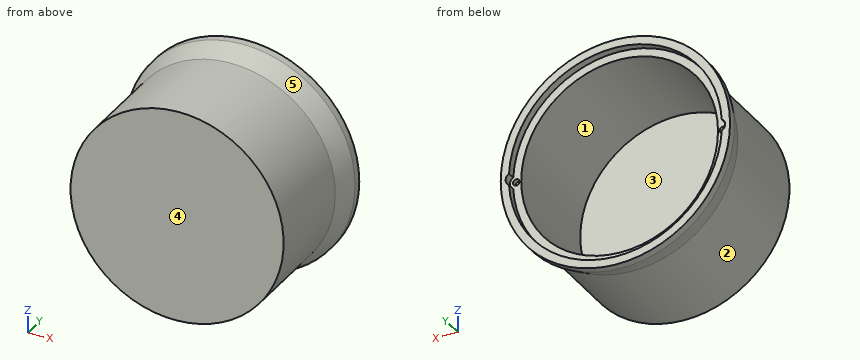
from build123d import *

# Parameters (mm, degrees)
SKETCH2_R          = 4
SKETCH2_R_2        = 2
CUT_EXTRUDE1_DEPTH = 125.761772992
SKETCH2_4_R        = 2
CUT_EXTRUDE3_DEPTH = 3


with BuildPart() as part:
    # Sketch1 → Revolve1 (revolve)
    with BuildSketch(Plane.XY, mode=Mode.PRIVATE) as revolve1_sk:
        Polygon((-70.5, 80), (-70.5, 75), (-65.5, 61.262612903), (-65.5, 0), (0, 0), (0, 5), (-60.5, 5), (-60.5, 75), (-65.5, 75), (-65.5, 80), align=None)
    revolve(revolve1_sk.sketch.rotate(Axis((0, 5, 0), (0, -1, 0)), 270), axis=Axis((0, 5, 0), (0, -1, 0)))

    # Sketch2 → Cut-Extrude1 (cut, through all)
    # profile 1 of 2: a face of its own
    with BuildSketch(Plane(origin=(0, 75, 0), x_dir=(1, 0, 0), z_dir=(0, 1, 0))):
        with Locations((-63.5, 0)):
            Circle(SKETCH2_R)
        with Locations((-63.5, 0)):
            Circle(SKETCH2_R_2, mode=Mode.SUBTRACT)
    # profile 2 of 2: a face of its own
    with BuildSketch(Plane(origin=(0, 75, 0), x_dir=(1, 0, 0), z_dir=(0, 1, 0))):
        with Locations((63.5, 0)):
            Circle(SKETCH2_R)
        with Locations((63.5, 0)):
            Circle(SKETCH2_R_2, mode=Mode.SUBTRACT)
    extrude(amount=CUT_EXTRUDE1_DEPTH, mode=Mode.SUBTRACT)

    # Sketch2_4 → Cut-Extrude3 (cut)
    with BuildSketch(Plane(origin=(0, 75, 0), x_dir=(1, 0, 0), z_dir=(0, 1, 0))):
        with Locations(Location((-63.5, 0, 0), (0, 0, 270))):
            Circle(SKETCH2_4_R)
        with Locations(Location((63.5, 0, 0), (0, 0, 270))):
            Circle(SKETCH2_4_R)
    extrude(amount=-CUT_EXTRUDE3_DEPTH, mode=Mode.SUBTRACT)


solid = part.part
Can you work these out from the model? Positions are in its coordinate system, mm. Face numbers are marked on the shaded views. A direction names the side the tool comes from. Coordinates: 2 decimals unless noted, no trailing zeros. Loops run counter-clockwise (first coordinate to the right, second up) from the corner with the lowest first, then second, coordinate; pieces in that order, holes last. Notation, with made-up numbers: M -20.75,62.25 L 29.25,62.25 A25 ccw 29.25,75.25 Z; hole C 30,36 d3. An arc over 180 degrees is marked long. Return JSON: item names as keys, results as strings. Group by question number.
Item 1: Thinking about a two-plate mould opening in X: for the marked faces 3, 4 and 5, which applies, released by +X, released by -X, zero draft, split by the parting line, or undercut?
Item 2: If I drill on L1, parallel to X at y = 74, z = 0; L2, parallel to X at y = 56, z = 0; L3, parallel to Y at x = -41.5, z = 46, over which ranges is the centre line in solid material (lowest first)? Write a range as from..to.
Item 3: Imagine slicing it at B-B (x = 0). Please give me the cut outline in (y, z).
Item 4: On a 3-axis mill with a long thin cutter (end or side, diameter ignored), from which of +Z, -Z, +X, -X, +Y, -Y can I reach the whole of each face in a straight line? I mean the marked faces 1 and 2. Say none if no direction works.
Item 5: Imagine slicing it at A-A (z = 0). Please give me the cut outline in (x, y), and give its area (3 significant figures).
Item 6: I'm going to push flat-ended pins straight in: pin 1 Ø1.2 at (x, z) = (64, 0) entering from +Y; pin 2 Ø4.5 at (x, z) = (63.5, 0) entering from +Y; pin 3 Ø12 at (x, z) = (-10, -18.5) entering from +Y. Where does each tip first touch, or does it pass through?
Item 7: Imagine slicing it at C-C (y = 54). Please give me the cut outline in (x, z), and give its area (3 significant figures).
Verdict:
{
 "1": {"face 3": "undercut", "face 4": "zero draft", "face 5": "split by the parting line"},
 "2": {"L1": "x = -70.14..-65.5, -61.5..-60.5, 60.5..61.5, 65.5..70.14", "L2": "x = -65.5..-60.5, 60.5..65.5", "L3": "y = 0..75"},
 "3": {"outline": "M 0,-65.5 L 61.26,-65.5 L 75,-70.5 L 80,-70.5 L 80,-65.5 L 75,-65.5 L 75,-60.5 L 5,-60.5 L 5,60.5 L 75,60.5 L 75,65.5 L 80,65.5 L 80,70.5 L 75,70.5 L 61.26,65.5 L 0,65.5 Z"},
 "4": {"face 1": "+Y", "face 2": "-Y"},
 "5": {"outline": "M -70.5,75 L -65.5,61.26 L -65.5,0 L 65.5,0 L 65.5,61.26 L 70.5,75 L 70.5,80 L 67.5,80 L 67.5,75 L 65.5,75 L 65.5,72 L 61.5,72 L 61.5,75 L 60.5,75 L 60.5,5 L -60.5,5 L -60.5,75 L -61.5,75 L -61.5,72 L -65.5,72 L -65.5,75 L -67.5,75 L -67.5,80 L -70.5,80 Z", "area": "1,430 mm^2"},
 "6": {"pin 1": "stops at y = 72", "pin 2": "stops at y = 75", "pin 3": "stops at y = 5"},
 "7": {"outline": "C 0,0 d131; hole C 0,0 d121", "area": "1,980 mm^2"}
}
